Design review of the part built by this model. Coordinates are the model's own, in mm. A direction names the side the tool comes from. Round coordinates to 2 decimals unless told otherwise and drop trailing zeros. Loops run counter-clockwise (first coordinate to the right, second up) from the corner with the lowest first, then second, coordinate; pieces in that order, holes last. Notation, with made-up numbers: (36, -10.75) -> (82, -10.75) arc R13 ccw to (82, -0.75) -> close; hole circle Ø4 at (-9, 71.5). An arc over 180 degrees is marked (long way). Answer as CSV lines item,"result". Start each with the question number.
(1) To check wall thickness, follow line 1 (X direction, y = 0, z = 0.5); line 2 (Z direction, x = -8.25, y = 0); line 3 (Y direction, x = -1.5, z = 2). State the ranges of each line that lie inside material, in increasing order. Write a range as from..to.
(2) For P1, Ø2, axis at x = 2, z = 4.5, coming from the +Y side; P2, Ø1.5, axis at x = -5.5, z = 1.5, coming from the -Y side; P3, Ø3, axis at y = -5.5, z = 4.5, coming from the +X side, all flat-tipped, find the tip position at first contact; note any pin that passes through.
(3) Take a section at B-B, the plane z = 2.25. Write out the cut boundary in (x, y).
(4) Draft analysis for pull direction Y (two halves, no side actions). For faces 3 (the face through (5, 0, 0)), 4 (the face through (-3.874, 0, 5)), 5 (the face through (10.48, 3.3, 3.13)), state which applies: +Y half, -Y half, draft (parallel to the pull), parting line (faces both ways), or undercut.
(5) Take a section at C-C, the plane x = 0. Write out the cut boundary in (y, z), and give its area (3 significant figures).
(6) Take a section at A-A, the plane y = 0. Write out the cut boundary in (x, z), and give its area (3 significant figures).
(7) Take a section at D-D, the plane x = 2.25. Write out the cut boundary in (y, z), and give its area (3 significant figures).
(8) Machinability: for faces 1 (the face through (5, 0, 6.35)), 2 (the face through (3.874, 0, 5)), which of the approach directions +Z, -Z, +X, -X, +Y, -Y give a long, thin tool a straight path to every point of the face, cutting with its end or side? Answer none if there is none.
from build123d import *

# Parameters (mm, degrees)
SKETCH1_R                           = 10.9855
SKETCH1_W                           = 7.747
SKETCH1_H                           = 7.747
BOSS_EXTRUDE1_DEPTH                 = 6.35
F_6_32_TAPPED_HOLE1_D               = 2.7051
F_6_32_TAPPED_HOLE1_DEPTH           = 7.112
F_6_32_TAPPED_HOLE1_ON_FACE_2_D     = 2.7051
F_6_32_TAPPED_HOLE1_ON_FACE_2_DEPTH = 7.112
F_6_32_TAPPED_HOLE2_D               = 2.7051
F_45_0_082_DIAMETER_HOLE1_D         = 2.0828


with BuildPart() as part:
    # Sketch1 → Boss-Extrude1 (new body)
    with BuildSketch(Plane.XY):
        Circle(SKETCH1_R)
        Rectangle(SKETCH1_W, SKETCH1_H, mode=Mode.SUBTRACT)
    extrude(amount=BOSS_EXTRUDE1_DEPTH)

    # #6-32 Tapped Hole1
    with Locations(Plane(origin=(10.9855, 0, 3.175), x_dir=(0, 0, 1), z_dir=(1, 0, 0))):
        with Locations((0, 0)):
            Hole(F_6_32_TAPPED_HOLE1_D / 2, depth=F_6_32_TAPPED_HOLE1_DEPTH)

    # #6-32 Tapped Hole1 on face 2
    with Locations(Plane(origin=(3.8735, 0, 3.175), x_dir=(0, 0, -1), z_dir=(-1, 0, 0))):
        with Locations((0, 0)):
            Hole(F_6_32_TAPPED_HOLE1_ON_FACE_2_D / 2, depth=F_6_32_TAPPED_HOLE1_ON_FACE_2_DEPTH)

    # #6-32 Tapped Hole2 (through all)
    with Locations(Plane(origin=(-3.8735, 0, 0), x_dir=(0, 0, -1), z_dir=(1, 0, 0))):
        with Locations((-3.175, 0)):
            Hole(F_6_32_TAPPED_HOLE2_D / 2)

    # #45 (0.082) Diameter Hole1 (through all)
    with Locations(Plane(origin=(0, 0, 0), x_dir=(-1, 0, 0), z_dir=(0, 0, -1))):
        with Locations((0, -7.4295), (0, 7.4295)):
            Hole(F_45_0_082_DIAMETER_HOLE1_D / 2)


solid = part.part
The answers:
1,line 1,"-10.99..-3.87, 3.87..10.99"
1,line 2,"0..1.82, 4.53..6.35"
1,line 3,"-10.88..-3.87, 3.87..10.88"
2,P1,"y = 10.94"
2,P2,"y = -9.91"
2,P3,"x = 10.23"
3,outline,"(-10.94, -0.99) arc R10.99 ccw to (10.94, -0.99) -> (3.87, -0.99) -> (3.87, -3.87) -> (-3.87, -3.87) -> (-3.87, -0.99) -> close; (-10.94, 0.99) -> (-3.87, 0.99) -> (-3.87, 3.87) -> (3.87, 3.87) -> (3.87, 0.99) -> (10.94, 0.99) arc R10.99 ccw to start; hole circle Ø2.08 at (0, -7.43); hole circle Ø2.08 at (0, 7.43)"
4,face 3,"draft"
4,face 4,"undercut"
4,face 5,"parting line"
5,outline,"(-10.99, 0) -> (-8.47, 0) -> (-8.47, 6.35) -> (-10.99, 6.35) -> close; (-6.39, 0) -> (-3.87, 0) -> (-3.87, 6.35) -> (-6.39, 6.35) -> close; (3.87, 0) -> (6.39, 0) -> (6.39, 6.35) -> (3.87, 6.35) -> close; (8.47, 0) -> (10.99, 0) -> (10.99, 6.35) -> (8.47, 6.35) -> close"
5,area,"63.9 mm²"
6,outline,"(-10.99, 0) -> (-3.87, 0) -> (-3.87, 1.82) -> (-10.99, 1.82) -> close; (-10.99, 4.53) -> (-3.87, 4.53) -> (-3.87, 6.35) -> (-10.99, 6.35) -> close; (3.87, 0) -> (10.99, 0) -> (10.99, 1.82) -> (3.87, 1.82) -> close; (3.87, 4.53) -> (10.99, 4.53) -> (10.99, 6.35) -> (3.87, 6.35) -> close"
6,area,"51.8 mm²"
7,outline,"(-10.75, 0) -> (-3.87, 0) -> (-3.87, 6.35) -> (-10.75, 6.35) -> close; (3.87, 0) -> (10.75, 0) -> (10.75, 6.35) -> (3.87, 6.35) -> close"
7,area,"87.4 mm²"
8,face 1,"+Z, +X, -X, +Y, -Y"
8,face 2,"+Z, -Z"
